Autodesk Inventor part; units mm, degrees
ref_plane "YZ Plane" through (0, 0, 0) normal (1, 0, 0) x (0, 1, 0)
ref_plane "XY Plane" through (0, 0, 0) normal (0, 0, 1) x (1, 0, 0)
sketch "Sketch1" plane through (0, 0, 0) normal (1, 0, 0) x (0, 1, 0)
  line L0 (0, 0) -> (11, 0)
  line L1 (11, 0) -> (11, -2.5)
  line L2 (11, -2.5) -> (8.5, -2.5)
  line L3 (8.5, -2.5) -> (8.5, -14.5)
  line L4 (8.5, -14.5) -> (7.5, -14.5)
  line L5 (7.5, -14.5) -> (7.5, -43)
  line L6 (7.5, -43) -> (5, -43)
  line L7 (5, -43) -> (5, -44.25)
  line L8 (5, -44.25) -> (7.5, -44.25)
  line L9 (7.5, -44.25) -> (7.5, -50.5)
  line L10 (7.5, -50.5) -> (6, -50.5)
  line L11 (6, -50.5) -> (6, -58.5)
  line L12 (6, -58.5) -> (5, -58.5)
  line L13 (5, -58.5) -> (5, -115.5)
  line L14 (5, -115.5) -> (0, -115.5)
  line L15 (0, -115.5) -> (0, 0)
  dimension "d0" = 5
  dimension "d1" = 6
  dimension "d2" = 7.5
  dimension "d3" = 5
  dimension "d4" = 8.5
  dimension "d5" = 7.5
  dimension "d6" = 11
  dimension "d7" = 2.5
  dimension "d8" = 12
  dimension "d9" = 1.25
  dimension "d10" = 6.25
  dimension "d12" = 57
  dimension "d13" = 65
  dimension "d14" = 28.5
revolve "Revolution1" add sketch "Sketch1" angle 360 about axis through (0, 0, -115.5) along (0, 0, 1)
sketch "Sketch2" plane through (0, 0, 0) normal (0, 0, 1) x (1, 0, 0)
  circle A0 centre (0, 10.64) radius 9
  arc A1 (-34.3908, -12.228) -> (34.3908, -12.228) centre (0, 0) ccw
  line L0 (0, 0) -> (118.8939, 0) construction
  line L1 (8.5595, 13.4212) -> (12.3892, 1.6344)
  circle A2 centre (0, 0) radius 5 construction
  line L2 (0, 0) -> (0, 32.7762) construction
  line L3 (14.4714, -0.7398) -> (33.3674, -9.7528)
  line L4 (-8.5595, 13.4212) -> (-12.3892, 1.6344)
  line L5 (-14.4714, -0.7398) -> (-33.3674, -9.7528)
  arc A3 (12.3892, 1.6344) -> (14.4714, -0.7398) centre (16.1935, 2.8705) ccw
  arc A4 (-14.4714, -0.7398) -> (-12.3892, 1.6344) centre (-16.1935, 2.8705) ccw
  arc A5 (34.3908, -12.228) -> (33.3674, -9.7528) centre (32.5064, -11.5579) ccw
  arc A6 (-33.3674, -9.7528) -> (-34.3908, -12.228) centre (-32.5064, -11.5579) ccw
  line L6 (0, 19.64) -> (56.14, 19.64) construction
  line L7 (0, -36.5) -> (89.4441, -36.5) construction
  point P0 (34.9542, -10.5096)
  point P1 (-34.9542, -10.5096)
  point P2 (-12.9203, 0)
  point P3 (12.9203, 0)
  dimension "d16" = 18
  dimension "d17" = 73
  dimension "d18" = 10.64
  dimension "d19" = 18
  dimension "d20" = 25.5
  dimension "d21" = 4
  dimension "d22" = 2
  dimension "d24" = 56.14
  dimension "d25" = 18
  dimension "d26" = 25.5
extrude "Extrusion1" add sketch "Sketch2" along normal blind 7
sketch "Sketch3" plane through (0, 0, 7) normal (0, 0, 1) x (1, 0, 0)
  arc A0 (8.5595, 13.4212) -> (-8.5595, 13.4212) centre (0, 10.64) ccw
  circle A1 centre (0, 10.64) radius 9
  point P0 (0, 0)
extrude "Extrusion2" add sketch "Sketch3" along normal blind 1.5
sketch "Sketch4" plane through (0, 10.64, 8.5) normal (0, 0, 1) x (1, 0, 0)
  circle A0 centre (0, 0) radius 5
  point P0 (0, -10.64)
  dimension "d31" = 10
extrude "Extrusion3" add sketch "Sketch4" along normal blind 15
sketch "Sketch5" plane through (0, 10.64, 23.5) normal (0, 0, 1) x (1, 0, 0)
  circle A0 centre (0, 0) radius 4.5
  circle A1 centre (0, 0) radius 9 construction
  point P0 (0, -10.64)
  dimension "d35" = 9
extrude "Extrusion4" add sketch "Sketch5" along normal blind 1.1
sketch "Sketch6" plane through (0, 10.64, 24.6) normal (0, 0, 1) x (1, 0, 0)
  circle A0 centre (0, 0) radius 5
  point P0 (0, -10.64)
  dimension "d38" = 10
extrude "Extrusion5" add sketch "Sketch6" along normal blind 1.6
chamfer "Chamfer1" distance 0.8 angle 45 1 edges at (-5, 10.64, 26.2) measured on face at (0.4847, 10.64, 26.2)
thread "Thread1"
ref_plane "Work Plane1" through (0, 7.5, -28.75) normal (0, 1, 0) x (-1, 0, 0)
sketch "Sketch7" plane through (0, 7.5, -28.75) normal (0, 1, 0) x (-1, 0, 0)
  line L0 (-8.5, 14.25) -> (8.5, 14.25) construction
  line L1 (0, 12.25) -> (0, 7.25) construction
  line L2 (-1.5, 12.25) -> (-1.5, 7.25)
  line L3 (1.5, 7.25) -> (1.5, 12.25)
  arc A0 (1.5, 12.25) -> (-1.5, 12.25) centre (0, 12.25) ccw
  arc A1 (-1.5, 7.25) -> (1.5, 7.25) centre (0, 7.25) ccw
  point P0 (0, 28.75)
  point P1 (0, 9.75)
  dimension "d46" = 1.5
  dimension "d47" = 5
  dimension "d48" = 0.5
extrude "Extrusion6" cut sketch "Sketch7" against normal blind 2
properties part number "Shaft"
Verification items for the finished model (mm, model axes). A direction names the side the tool comes from. Give positions to 0.01 mm unless a question says otherwise; leave off trailing zeros. Order: outer loops, then holes, each group sorted by start corner. A loop starts at its lowest first (then second) coordinate and runs counter-clockwise, first axis right, second up. Notation, with made-up numbers: (50.25, 49.5) - (101.25, 49.5) arc R25 ccw to (101.25, 86.5) - close; hole circle Ø6 at (80.25, 13). An arc over 180 degrees is marked (long way). Answer as CSV lines item,"result". Start each with the question number.
Item 1: Section check D-D, the plane z = -32.5. Record the boundary of the cut face in (x, y).
Item 2: Mould release check, pull along Z, two halves, no side actions. Record for faces 4 (the face through (-6, 2, -50.5)), 5 (the face through (-4.88, -1.08, -43.63)), 6 (the face through (-4.88, -1.08, -87.4)): released by +Z, released by -Z, zero draft, split by the parting line, or undercut.
Item 3: Section check A-A, the plane z = 3.5. Record the boundary of the cut face in (x, y), plus the area to 3 significant figures.
Item 4: Section check B-B, the plane x = -24. Record the boundary of the cut face in (y, z), plus the area to 3 significant figures.
Item 5: Access from +Z, -Z, +X, -X, +Y, -Y to the whole of each face (thin tool, end or side, straight path). Record for faces 1 (the face through (-0.651, 5.683, 15.895)), 2 (the face through (-2, 15, 23.5)), 3 (the face through (8.1, 3.2, -2.5)).
Item 6: Section check C-C, the plane y = -20. Record the boundary of the cut face in (x, z).
Item 7: Gauge pin test, flat ends, axial feed: pin 1 (25 mm diameter, centred on x = 4, y = -22.5, fed in from +Z); pin 2 (1.5 mm diameter, centred on y = 6, z = -20, fed in from +X); pin 3 (4 mm diameter, centred on x = 23.5, y = -26, fed in from -Z). Record the tip position at first contact, or that the pin passes through.
Item 8: Material ranges on L1, parallel to Z at x = -4.5, y = 3; L2, parallel to Z at x = -18.5, y = -11; L3, parallel to Y at x = 4.5, z = -17.5, recorded low to high.
Filled in:
1,outline,"circle Ø15 at (0, 0)"
2,face 4,"released by -Z"
2,face 5,"undercut"
2,face 6,"zero draft"
3,outline,"(-34.39, -12.23) arc R36.5 ccw to (34.39, -12.23) arc R2 ccw to (33.37, -9.75) - (14.47, -0.74) arc R4 cw to (12.39, 1.63) - (8.56, 13.42) arc R9 ccw to (-8.56, 13.42) - (-12.39, 1.63) arc R4 cw to (-14.47, -0.74) - (-33.37, -9.75) arc R2 ccw to start"
3,area,"2,210 mm^2"
4,outline,"(-27.5, 0) - (-5.28, 0) - (-5.28, 7) - (-27.5, 7) - close"
4,area,"156 mm^2"
5,face 1,"+Z"
5,face 2,"none"
5,face 3,"-Z"
6,outline,"(-30.53, 0) - (30.53, 0) - (30.53, 7) - (-30.53, 7) - close"
7,pin 1,"z = 7"
7,pin 2,"x = 5.36"
7,pin 3,"z = 0"
8,L1,"-58.5 to -44.25, -43 to 8.5"
8,L2,"0 to 7"
8,L3,"-6 to 6"
